Job drawing, mm, ordinate dimensions from the low corner. One solid piece. A direction names the side the tool comes from. Give positions to 0.01 mm unless a question says otherwise; leave off trailing zeros. Order: outer loops, then holes, each group sorted by start corner. A loop starts at its lowest first (then second) coordinate and runs counter-clockwise, first axis right, second up. Notation, with made-up numbers: M 35.5,1 L 66.5,1 A5 ccw 66.5,7 Z; hole C 79.25,77.5 d6. An arc over 180 degrees is marked long. One line per question, with ' | ' between items.
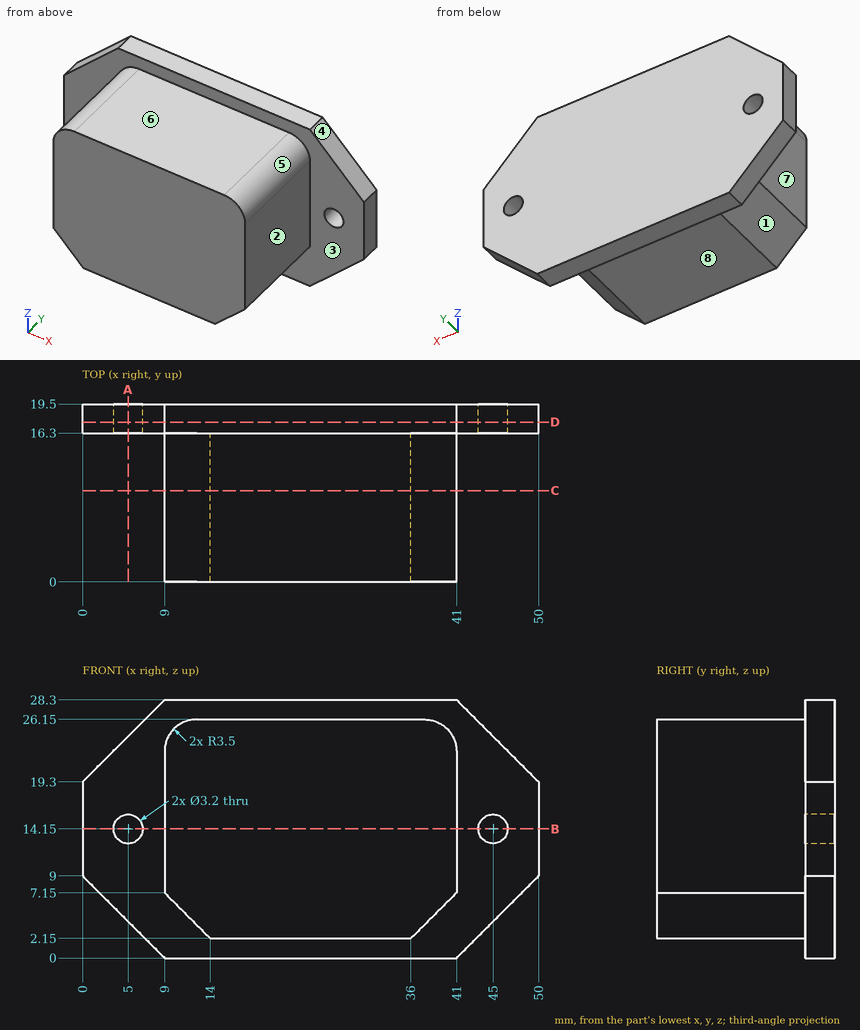
1. Slice it at A-A on x = 5. Give the cut face in (y, z), then the cut area to 3 significant figures.
Worked out:
outline: M 16.3,4 L 19.5,4 L 19.5,12.55 L 16.3,12.55 Z; M 16.3,15.75 L 19.5,15.75 L 19.5,24.3 L 16.3,24.3 Z | area: 54.7 mm2
2. Slice it at B-B on z = 14.15. Give the cut face in (x, y), then the cut area to 3 significant figures.
Worked out:
outline: M 0,16.3 L 3.4,16.3 L 3.4,19.5 L 0,19.5 Z; M 6.6,16.3 L 9,16.3 L 9,0 L 41,0 L 41,16.3 L 43.4,16.3 L 43.4,19.5 L 6.6,19.5 Z; M 46.6,16.3 L 50,16.3 L 50,19.5 L 46.6,19.5 Z | area: 661 mm2
3. Slice it at D-D on y = 17.5. Give the cut face in (x, z).
Worked out:
outline: M 0,9 L 9,0 L 41,0 L 50,9 L 50,19.3 L 41,28.3 L 9,28.3 L 0,19.3 Z; hole C 5,14.15 d3.2; hole C 45,14.15 d3.2
4. Tool access for the marked faces 1, 2, 3, 4 and 5: list every direction of +Z, -Z, +X, -X, +Y, -Y with a clear straight run to the whole face (end or side of a thin tool).
Worked out:
face 1: -Z, -X, -Y | face 2: +Z, -Z, +X, -Y | face 3: -Y | face 4: +Z, +X, +Y, -Y | face 5: +Z, +X, -Y
5. Probe L1, parallel to X at y = 17.9, z = 14.15; L2, parallel to Z at x = 32.5, y = 6.75; L3, parallel to Y at x = 20, z = 27.25. List the from-to ranges inside material, lowest first. Write a range as from..to.
Worked out:
L1: x = 0..3.4, 6.6..43.4, 46.6..50 | L2: z = 2.15..26.15 | L3: y = 16.3..19.5
6. Drop flat-ended pins along their axis: pin 1 (2 mm diameter, centred on x = 37.5, y = 14, fed in from +Z); pin 2 (7.5 mm diameter, centred on y = 7, z = 17.5, fed in from +X); pin 3 (4.5 mm diameter, centred on y = 10.5, z = 11.5, fed in from -X); pin 4 (2 mm diameter, centred on x = 10.5, z = 22, fed in from -Y). Give the stop position or say it passes through.
Worked out:
pin 1: stops at z = 26.15 | pin 2: stops at x = 41 | pin 3: stops at x = 9 | pin 4: stops at y = 0
7. Mould opens along Z. For the marked faces 6, 7 and 8 say: released by +Z, released by -Z, zero draft, split by the parting line, or undercut.
Worked out:
face 6: released by +Z | face 7: zero draft | face 8: released by -Z
8. Slice it at C-C on y = 10. Give the cut face in (x, z), then the cut area to 3 significant figures.
Worked out:
outline: M 9,7.15 L 14,2.15 L 36,2.15 L 41,7.15 L 41,22.65 A3.5 ccw 37.5,26.15 L 12.5,26.15 A3.5 ccw 9,22.65 Z | area: 738 mm2
